from build123d import *

# Parameters (mm, degrees)
F0_R     = 1.6
F1_DEPTH = 1.5
F3_DEPTH = 1.501


with BuildPart() as f1:
    # F0 (on Top) → F1 (new body)
    with BuildSketch(Plane.XY):
        with BuildLine():
            ThreePointArc((12.068019, 18.431981), (0, 13.433243), (-12.068019, 18.431981))
            ThreePointArc((-12.068019, 18.431981), (-18.431981, 18.431981), (-18.431981, 12.068019))
            ThreePointArc((-18.431981, 12.068019), (-13.433243, 0), (-18.431981, -12.068019))
            ThreePointArc((-18.431981, -12.068019), (-18.431981, -18.431981), (-12.068019, -18.431981))
            ThreePointArc((-12.068019, -18.431981), (0, -13.433243), (12.068019, -18.431981))
            ThreePointArc((12.068019, -18.431981), (18.431981, -18.431981), (18.431981, -12.068019))
            ThreePointArc((18.431981, -12.068019), (13.433243, 0), (18.431981, 12.068019))
            ThreePointArc((18.431981, 12.068019), (18.431981, 18.431981), (12.068019, 18.431981))
        make_face()
        with Locations((-15.25, -15.25)):
            Circle(F0_R, mode=Mode.SUBTRACT)
        with Locations((15.25, -15.25)):
            Circle(F0_R, mode=Mode.SUBTRACT)
        with Locations((-15.25, 15.25)):
            Circle(F0_R, mode=Mode.SUBTRACT)
        with Locations((15.25, 15.25)):
            Circle(F0_R, mode=Mode.SUBTRACT)
    extrude(amount=F1_DEPTH)

    # F2 (on face) → F3 (cut, through all)
    with BuildSketch(Plane.XY.offset(1.5)):
        with BuildLine():
            Line((-4, 2), (-4, 10))
            ThreePointArc((-4, 10), (-5, 11), (-6, 10))
            Line((-6, 10), (-6, 2))
            ThreePointArc((-6, 2), (-5, 1), (-4, 2))
        make_face()
        with BuildLine():
            ThreePointArc((6, 10), (5, 11), (4, 10))
            Line((4, 10), (4, 2))
            ThreePointArc((4, 2), (5, 1), (6, 2))
            Line((6, 2), (6, 10))
        make_face()
        with BuildLine():
            Line((-4, -10), (-4, -2))
            ThreePointArc((-4, -2), (-5, -1), (-6, -2))
            Line((-6, -2), (-6, -10))
            ThreePointArc((-6, -10), (-5, -11), (-4, -10))
        make_face()
        with BuildLine():
            ThreePointArc((6, -2), (5, -1), (4, -2))
            Line((4, -2), (4, -10))
            ThreePointArc((4, -10), (5, -11), (6, -10))
            Line((6, -10), (6, -2))
        make_face()
        with BuildLine():
            Line((-9, 2), (-9, 10))
            ThreePointArc((-9, 10), (-10, 11), (-11, 10))
            Line((-11, 10), (-11, 2))
            ThreePointArc((-11, 2), (-10, 1), (-9, 2))
        make_face()
        with BuildLine():
            Line((-9, -10), (-9, -2))
            ThreePointArc((-9, -2), (-10, -1), (-11, -2))
            Line((-11, -2), (-11, -10))
            ThreePointArc((-11, -10), (-10, -11), (-9, -10))
        make_face()
        with BuildLine():
            ThreePointArc((11, -2), (10, -1), (9, -2))
            Line((9, -2), (9, -10))
            ThreePointArc((9, -10), (10, -11), (11, -10))
            Line((11, -10), (11, -2))
        make_face()
        with BuildLine():
            Line((9, 10), (9, 2))
            ThreePointArc((9, 2), (10, 1), (11, 2))
            Line((11, 2), (11, 10))
            ThreePointArc((11, 10), (10, 11), (9, 10))
        make_face()
    extrude(amount=-F3_DEPTH, mode=Mode.SUBTRACT)


solid = f1.part
The listing builds one solid part. Answer for the finished solid, in the listing's coordinates (mm). A direction names the side the tool comes from. Coordinates: 2 decimals unless noted, no trailing zeros. Loops run counter-clockwise (first coordinate to the right, second up) from the corner with the lowest first, then second, coordinate; pieces in that order, holes last.
1) Find section D-D on y = 7. Write down the section's boundary in (x, z).
2) Find section C-C on x = 15.25. Write down the section's boundary in (y, z).
3) A tool of negligible diameter and unlimited length cuts with its end or side. For faces 4 (the face through (-4, 6, 1)), 5 (the face through (-13.434, 0.188, 0.74)), from which of +Z, -Z, +X, -X, +Y, -Y can it reach the whole face along a straight path? Write none if from no direction.
4) Find section B-B on x = -10. Write down the section's boundary in (y, z).
5) Flat-ended cylindrical pins translate along their axes: pin 1 Ø3.5 at (x, y) = (15.25, 15.25) entering from +Z; pin 2 Ø0.8 at (y, z) = (4.5, 1) entering from +X; pin 3 Ø1.9 at (x, y) = (-15.25, -15.25) entering from -Z; pin 4 Ø0.8 at (y, z) = (7, 1) entering from -X. Find the tip coordinate at first contact, or state that the pin passes through.
6) Find section A-A on y = -1.5. Write down the section's boundary in (x, z), then the cut area to 3 significant figures.
7) Determine the mould class of faces 1 (the face through (4, -6, 1)), 2 (the face through (0, 0, 1.5)), 3 (the face through (-0.188, -13.434, 0.74)) for opening direction Y: pulls with the +Y half, pulls with the -Y half, needs draft (parallel to the pull), parting line crosses it, or undercut.
8) Find the intervals of material crossed by L1, parallel to Y at x = 15.25, z = 1.15; L2, parallel to X at y = 4, z = 1.4; L3, parallel to Y at x = 5, z = 1.4, in increasing order.
Values:
1. outline: (-14.93, 0) - (-11, 0) - (-11, 1.5) - (-14.93, 1.5) - close; (-9, 0) - (-6, 0) - (-6, 1.5) - (-9, 1.5) - close; (-4, 0) - (4, 0) - (4, 1.5) - (-4, 1.5) - close; (6, 0) - (9, 0) - (9, 1.5) - (6, 1.5) - close; (11, 0) - (14.93, 0) - (14.93, 1.5) - (11, 1.5) - close
2. outline: (-19.75, 0) - (-16.85, 0) - (-16.85, 1.5) - (-19.75, 1.5) - close; (-13.65, 0) - (-7.66, 0) - (-7.66, 1.5) - (-13.65, 1.5) - close; (7.66, 0) - (13.65, 0) - (13.65, 1.5) - (7.66, 1.5) - close; (16.85, 0) - (19.75, 0) - (19.75, 1.5) - (16.85, 1.5) - close
3. face 4: +Z, -Z
3. face 5: +Z, -Z, -X
4. outline: (-16.67, 0) - (-11, 0) - (-11, 1.5) - (-16.67, 1.5) - close; (-1, 0) - (1, 0) - (1, 1.5) - (-1, 1.5) - close; (11, 0) - (16.67, 0) - (16.67, 1.5) - (11, 1.5) - close
5. pin 1: stops at z = 1.5
5. pin 2: stops at x = 14.15
5. pin 3: passes through
5. pin 4: stops at x = -15.12
6. outline: (-13.5, 0) - (-10.87, 0) - (-10.87, 1.5) - (-13.5, 1.5) - close; (-9.13, 0) - (-5.87, 0) - (-5.87, 1.5) - (-9.13, 1.5) - close; (-4.13, 0) - (4.13, 0) - (4.13, 1.5) - (-4.13, 1.5) - close; (5.87, 0) - (9.13, 0) - (9.13, 1.5) - (5.87, 1.5) - close; (10.87, 0) - (13.5, 0) - (13.5, 1.5) - (10.87, 1.5) - close
6. area: 30.1 mm2
7. face 1: undercut
7. face 2: needs draft
7. face 3: pulls with the -Y half
8. L1: y = -19.75 to -16.85, -13.65 to -7.66, 7.66 to 13.65, 16.85 to 19.75
8. L2: x = -13.91 to -11, -9 to -6, -4 to 4, 6 to 9, 11 to 13.91
8. L3: y = -14.18 to -11, -1 to 1, 11 to 14.18
